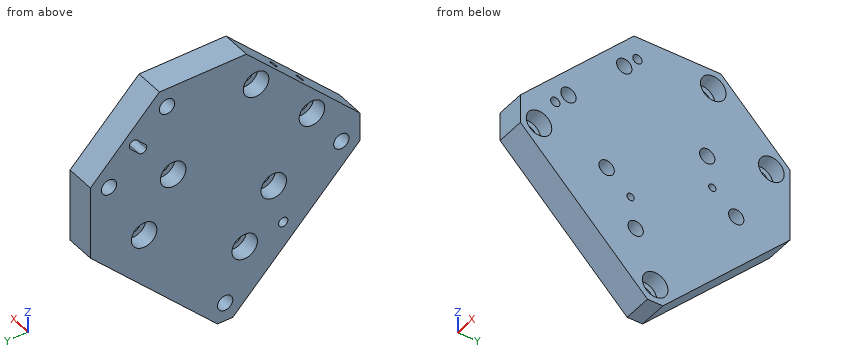
Autodesk Inventor part; units mm, degrees
ref_plane "YZ Plane" through (0, 0, 0) normal (1, 0, 0) x (0, 1, 0)
ref_plane "XZ Plane" through (0, 0, 0) normal (0, 1, 0) x (-1, 0, 0)
ref_plane "XY Plane" through (0, 0, 0) normal (0, 0, 1) x (1, 0, 0)
sketch "Sketch4" plane through (0, 0, 0) normal (1, 0, 0) x (0, 1, 0)
  line L0 (-56.119, -133.197) -> (-1.4327, -78.5108)
  line L1 (-68.5481, -17.197) -> (-117.4327, -66.0816)
  line L2 (-117.4327, -66.0816) -> (-117.4327, -78.5108)
  line L3 (-72.7358, -32.6985) -> (-96.7775, -56.7401) construction
  line L4 (-68.5481, -17.197) -> (-31.119, -17.197)
  line L5 (-1.4327, -78.5108) -> (-1.4327, -46.8833)
  line L6 (-1.4327, -46.8833) -> (-31.119, -17.197)
  line L7 (-56.119, -133.197) -> (-62.7464, -133.197)
  line L8 (-117.4327, -78.5108) -> (-62.7464, -133.197)
  circle A0 centre (-72.7358, -32.6985) radius 2.4585
  circle A1 centre (-96.7775, -56.7401) radius 2.4585
  point P0 (0, 0)
  point P1 (-59.4327, -125.197)
  point P2 (-34.4327, -25.197)
  point P3 (-9.4327, -50.197)
  point P4 (-109.4327, -75.197)
  dimension "d6" = 8
  dimension "d8" = 135
  dimension "d10" = 135
  dimension "d11" = 135
  dimension "d13" = 8
  dimension "d14" = 8
  dimension "d15" = 8
  dimension "d18" = 8
  dimension "d19" = 8
  dimension "d105" = 135
  dimension "d106" = 8
  dimension "d107" = 8
extrude "Extrusion2" add sketch "Sketch4" along normal blind 12.5 contours L7 L8 L2 L1 L4 L6 L5 L0 | A0 | A1
sketch "Sketch9" plane through (0, 0, 0) normal (-1, 0, 0) x (0, 0, 1)
  circle A0 centre (-78.6225, -24.5414) radius 2.5
  circle A1 centre (-56.9775, -37.0382) radius 2.5
  circle A2 centre (-103.6161, -67.8315) radius 2.5
  circle A3 centre (-81.9711, -80.3283) radius 2.5
  circle A4 centre (-32.6985, -72.7358) radius 2.4585
  circle A5 centre (-56.7401, -96.7775) radius 2.4585
hole "M6ClearanceToPayload" at (0, -24.5414, -78.6225) at (0, -37.0382, -56.9775) at (0, -80.3283, -81.9711) at (0, -67.8315, -103.6161) at (0, -96.7775, -56.7401) at (0, -72.7358, -32.6985) direction (1, 0, 0) diameter 6.6 end through all counterbore diameter 11 counterbore depth 6.8
sketch "Sketch11" plane through (12.5, 0, 0) normal (1, 0, 0) x (0, 0, -1)
  circle A0 centre (70.1368, -34.8372) radius 1.6002
  circle A1 centre (90.4568, -70.0325) radius 1.6002
hole "1/8\" dowel holes" at (12.5, -34.8372, -70.1368) at (12.5, -70.0325, -90.4568) direction (-1, 0, 0) diameter 3.175 depth 3.5 tip angle 118
sketch "Sketch12" plane through (12.5, 0, 0) normal (1, 0, 0) x (0, 0, -1)
  line L0 (63.8112, -101.0201) -> (60.9827, -103.8485)
  circle A0 centre (27.0416, -67.079) radius 2
  line L1 (61.6898, -104.5556) -> (60.2756, -103.1414)
  line L2 (63.104, -100.313) -> (64.5183, -101.7272)
  point P0 (27.0416, -67.079)
  point P1 (62.3969, -102.4343)
  point P2 (27.0416, -67.079)
hole "4P6 dowel holes" at (12.5, -67.079, -27.0416) at (12.5, -102.4343, -62.3969) direction (-1, 0, 0) diameter 4 depth 8 tip angle 118
sketch "Sketch8" plane through (12.5, 0, 0) normal (1, 0, 0) x (0, 0, -1)
  point P0 (25.197, -34.4327)
  point P1 (50.197, -9.4327)
  point P2 (125.197, -59.4327)
  point P3 (75.197, -109.4327)
hole "M6ClearanceToSubstrate" at (12.5, -34.4327, -25.197) at (12.5, -9.4327, -50.197) at (12.5, -59.4327, -125.197) at (12.5, -109.4327, -75.197) direction (-1, 0, 0) diameter 6.6 end through all counterbore diameter 11 counterbore depth 6.8
sketch "Sketch13" plane through (0, 0, 0) normal (-1, 0, 0) x (0, 0, 1)
  circle A0 centre (-50.197, -9.4327) radius 3.3
  circle A1 centre (-25.197, -34.4327) radius 3.3
  line L0 (-50.197, -9.4327) -> (-25.197, -34.4327) construction
  circle A2 centre (-125.197, -59.4327) radius 3.3
  circle A3 centre (-75.197, -109.4327) radius 3.3
  line L1 (-125.197, -59.4327) -> (-75.197, -109.4327) construction
  line L2 (-37.697, -21.9327) -> (-100.197, -84.4327)
  line L3 (-35.9293, -20.1649) -> (-39.4648, -23.7004) construction
  line L4 (-37.3435, -18.7507) -> (-40.879, -22.2862)
  line L5 (-38.0506, -25.1147) -> (-34.5151, -21.5791)
  arc A4 (-34.5151, -21.5791) -> (-37.3435, -18.7507) centre (-35.9293, -20.1649) ccw
  arc A5 (-40.879, -22.2862) -> (-38.0506, -25.1147) centre (-39.4648, -23.7004) ccw
  dimension "d78" = 2.5
  dimension "d79" = 4
hole "4H7 location holes" at (0, -20.1649, -35.9293) at (0, -23.7004, -39.4648) at (0, -84.4327, -100.197) direction (1, 0, 0) diameter 4 depth 8
extrude "Extrusion3" cut sketch "Sketch13" against normal blind 8 contours A4 L5 A5 L4
sketch "Sketch16" plane through (0, -117.4327, -66.0816) normal (0, -0.7071, 0.7071) x (1, 0, 0)
  line L0 (0, 21.2109) -> (12.5, 21.2109) construction
  line L1 (0, 55.2109) -> (11.8351, 55.2109) construction
  line L2 (6.5, 21.2109) -> (6.5, 55.2109) construction
  line L3 (12.5, 69.1332) -> (12.5, 0) construction
  line L4 (1.6198, 38.2109) -> (11.3802, 38.2109)
  line L5 (6.8, 49.7109) -> (6.8, 60.7109)
  line L6 (6.8, 15.7109) -> (6.8, 26.7109)
  line L7 (0, 49.7109) -> (0, 60.7109)
  line L8 (0, 15.7109) -> (0, 26.7109)
  point P0 (6.5, 38.2109)
  point P1 (6.5, 30.2109)
  point P2 (6.5, 46.2109)
  point P3 (6.8, 21.2109)
  dimension "d96" = 6
  dimension "d97" = 16
hole "Hole11" at (6.5, -96.0704, -44.7193) at (6.5, -84.7567, -33.4056) direction (0, 0.7071, -0.7071) diameter 3.242 depth 11.8 tip angle 118
equation "\"d6\" = border"
equation "\"d10\" = d8"
equation "\"d11\" = d8"
equation "\"d105\" = d10"
equation "\"d64\" = thorlabsPinDiameter"
equation "\"border\" = 8"
equation "\"thorlabsPinDiameter\" = 3.175"
properties part number "FAB-OX0003" material "Aluminum 6061"
Source: CAD feature listing. Evaluate the final solid. Frame: model axes, mm. Coordinates: 2 decimals unless noted, no trailing zeros. Loops run counter-clockwise (first coordinate to the right, second up) from the corner with the lowest first, then second, coordinate; pieces in that order, holes last. Notation, with made-up numbers: (-16, -3) - (35, -3) arc R12 cw to (35, 17) - close; hole circle Ø9 at (58.5, -30). An arc over 180 degrees is marked (long way). Return JSON: item names as keys, results as strings.
Q1. Section B-B, the plane z = -57.5. Return loops of the section in (x, y), plus the area to 3 significant figures.
Results:
{"outline": "(0, -108.85) - (12.5, -108.85) - (12.5, -99.99) - (6.8, -99.99) - (6.8, -102.22) - (0, -102.22) - close; (0, -91.33) - (6.8, -91.33) - (6.8, -93.57) - (12.5, -93.57) - (12.5, -40.3) - (6.8, -40.3) - (6.8, -42.51) - (0, -42.51) - close; (0, -31.56) - (6.8, -31.56) - (6.8, -33.78) - (12.5, -33.78) - (12.5, -1.43) - (0, -1.43) - close", "area": "1,120 mm2"}
Q2. Section C-C, the plane z = -95. Return loops of the section in (x, y).
Results:
{"outline": "(0, -100.94) - (12.5, -100.94) - (12.5, -17.92) - (0, -17.92) - close"}
Q3. Section A-A, the plane x = 1.75. Give the number of separate pieces and of enclosed holes in the cut face, plus the area to 3 significant figures.
Results:
{"separate pieces": "1", "enclosed holes": "12", "area": "8,080 mm2"}
Q4. Contact query for flat-ended pins moving along their axis: P1, Ø5.5, axis at y = -72.5, z = -31.5, coming from the -X side; P2, Ø1, axis at x = 9, y = -102.5, coming from the -Z side; P3, Ø4, axis at x = 7.5, z = -40, coming from the +Y side. Output: stop coordinate, or through.
Results:
{"P1": "x = 6.8", "P2": "z = -93.94", "P3": "y = -6.32"}
Q5. Material intervals for line 1 along Z through (x, y) = (6.25, -38); line 2 along Z through (x, y) = (7.75, -70.5); line 3 along Y through (x, z) = (4.5, -36), sorted ascending.
Results:
{"line 1": "-115.08 to -62.39, -51.56 to -29.38, -21.01 to -17.2", "line 2": "-125.44 to -105.56, -101.67 to -35.13, -30.27 to -19.15", "line 3": "-87.35 to -77.13, -68.34 to -23.06, -18.17 to -12.32"}
